Build history of the part. All positions in model axes, mm. Face numbers are marked on the shaded views. Give positions to 0.01 mm unless a question says otherwise; leave off trailing zeros. Write each loop counter-clockwise with the first axis right and the second up, starting at its lowest first coordinate (ties: lowest second). Pieces come first, ordered by that corner, then holes. Notation, with made-up numbers: (49, 58) -> (56, 58) arc R21 ccw to (56, 73) -> close; hole circle Ø10 at (70, -20). An arc over 180 degrees is marked (long way). Put each result on its own line as item: value.
from build123d import *

# Parameters (mm, degrees)
ESBO_O1_R                     = 2.25
RESSALTO_EXTRUS_O1_DEPTH      = 4
RESSALTO_EXTRUS_O2_DEPTH      = 10
RESSALTO_EXTRUS_O2_DEPTH_BACK = 4
ESBO_O2_W                     = 10
ESBO_O2_H                     = 20
ESBO_O2_R                     = 1.5
ESBO_O2_W_2                   = 3
FILETE1_R                     = 3
FILETE2_R                     = 3
FILETE3_R                     = 10
FILETE4_R                     = 10
FILETE6_R                     = 5
FILETE7_R                     = 5
FILETE8_R                     = 5


# Some blends are built 0.0001 mm under size
with BuildPart() as part:
    # Esboço1 → Ressalto-extrusão1 (new body)
    with BuildSketch(Plane.XY):
        with BuildLine():
            Line((30, 15.55), (30, 30.45))
            Line((30, 30.45), (30, 45.35))
            ThreePointArc((30, 45.35), (28.681980515, 48.531980515), (25.5, 49.85))
            Line((25.5, 49.85), (24.5, 49.85))
            Line((24.5, 49.85), (-26.5, 49.85))
            ThreePointArc((-26.5, 49.85), (-29.681980515, 48.531980515), (-31, 45.35))
            Line((-31, 45.35), (-31, 30.45))
            Line((-31, 30.45), (-31, 15.55))
            ThreePointArc((-31, 15.55), (-29.681980515, 12.368019485), (-26.5, 11.05))
            Line((-26.5, 11.05), (25.5, 11.05))
            ThreePointArc((25.5, 11.05), (28.681980515, 12.368019485), (30, 15.55))
        make_face()
        with Locations((-24.8, 25.45)):
            Circle(ESBO_O1_R, mode=Mode.SUBTRACT)
        with Locations((23.8, 25.45)):
            Circle(ESBO_O1_R, mode=Mode.SUBTRACT)
        with Locations((-24.8, 35.45)):
            Circle(ESBO_O1_R, mode=Mode.SUBTRACT)
        Polygon((27, 31.05), (27, 30.45), (27, 29.85), (20, 29.85), (20, 20.45), (-21, 20.45), (-21, 29.85), (-28, 29.85), (-28, 31.05), (-21, 31.05), (-21, 40.45), (20, 40.45), (20, 31.05), align=None, mode=Mode.SUBTRACT)
        with Locations((23.8, 35.45)):
            Circle(ESBO_O1_R, mode=Mode.SUBTRACT)
    extrude(amount=RESSALTO_EXTRUS_O1_DEPTH)

    # Esboço2 → Ressalto-extrusão2 (add, two sides: drawn at the far end of the back side and taken through both)
    # profile 1 of 5: a face of its own
    with BuildSketch(Plane.XY.offset(4).offset(-RESSALTO_EXTRUS_O2_DEPTH_BACK)):
        with Locations((-0.6, 59.85)):
            Rectangle(ESBO_O2_W, ESBO_O2_H)
        with Locations((-1.6, 54.35)):
            Circle(ESBO_O2_R, mode=Mode.SUBTRACT)
        with Locations((-1.6, 63.85)):
            Circle(ESBO_O2_R, mode=Mode.SUBTRACT)
    # profile 2 of 5: a face of its own
    with BuildSketch(Plane.XY.offset(4).offset(-RESSALTO_EXTRUS_O2_DEPTH_BACK)):
        with Locations((5.9, 59.85)):
            Rectangle(ESBO_O2_W_2, ESBO_O2_H)
    # profile 3 of 5: a face of its own
    with BuildSketch(Plane.XY.offset(4).offset(-RESSALTO_EXTRUS_O2_DEPTH_BACK)):
        Polygon((30, 32.45), (30, 30.45), (30, 28.45), (55, 28.45), (55, 32.45), align=None)
    # profile 4 of 5: a face of its own
    with BuildSketch(Plane.XY.offset(4).offset(-RESSALTO_EXTRUS_O2_DEPTH_BACK)):
        with Locations((-0.6, 1.05)):
            Rectangle(ESBO_O2_W, ESBO_O2_H)
        with Locations((-1.6, -2.95)):
            Circle(ESBO_O2_R, mode=Mode.SUBTRACT)
        with Locations((-1.6, 6.55)):
            Circle(ESBO_O2_R, mode=Mode.SUBTRACT)
    # profile 5 of 5: a face of its own
    with BuildSketch(Plane.XY.offset(4).offset(-RESSALTO_EXTRUS_O2_DEPTH_BACK)):
        with Locations((5.9, 1.05)):
            Rectangle(ESBO_O2_W_2, ESBO_O2_H)
    extrude(amount=RESSALTO_EXTRUS_O2_DEPTH + RESSALTO_EXTRUS_O2_DEPTH_BACK)

    # Filete1
    filete1_edges = [part.edges().sort_by_distance(p)[0] for p in [
        (30, 30.45, 4),
    ]]
    fillet(filete1_edges, radius=FILETE1_R - 0.0001)  # a hair under: the kernel refuses the full size

    # Filete2
    filete2_edges = [part.edges().sort_by_distance(p)[0] for p in [
        (30, 30.45, 14),
    ]]
    fillet(filete2_edges, radius=FILETE2_R)

    # Filete3
    # the kernel refuses this fillet: 10 mm, written as the material it adds along each edge
    with BuildSketch(Plane(origin=(-5.6, 11.05, 4), x_dir=(0, 1, 0), z_dir=(1, 0, 0))) as filete3_piece_1:
        with BuildLine():
            CenterArc((10, 9.981983771), FILETE3_R, 180, 86.560187232)
            Line((0, 9.981983771), (0, 0))
            Line((0, 0), (9.4, 0))
        make_face()
    extrude(amount=13)

    # Filete4
    # the kernel refuses this fillet: 10 mm, written as the material it adds along each edge
    with BuildSketch(Plane(origin=(-5.6, 49.85, 4), x_dir=(0, -1, 0), z_dir=(1, 0, 0))) as filete4_piece_1:
        with BuildLine():
            CenterArc((10, -9.981983771), FILETE4_R, 93.439812768, 86.560187232)
            Line((0, -9.981983771), (0, 0))
            Line((0, 0), (9.4, 0))
        make_face()
    extrude(amount=13)

    # Filete6
    # the kernel refuses this fillet: 5 mm, written as the material it takes off along each edge
    with BuildSketch(Plane(origin=(-18.1, 69.85, 0), x_dir=(0, -1, 0), z_dir=(1, 0, 0))) as filete6_piece_1:
        with BuildLine():
            CenterArc((FILETE6_R, -FILETE6_R), FILETE6_R, 90, 90)
            Line((0, -FILETE6_R), (0, 0))
            Line((0, 0), (FILETE6_R, 0))
        make_face()
    extrude(amount=38, mode=Mode.SUBTRACT)

    # Filete7
    # the kernel refuses this fillet: 5 mm, written as the material it takes off along each edge
    with BuildSketch(Plane(origin=(19.9, -8.95, 0), x_dir=(0, 1, 0), z_dir=(-1, 0, 0))) as filete7_piece_1:
        with BuildLine():
            CenterArc((FILETE7_R, -FILETE7_R), FILETE7_R, 90, 90)
            Line((0, -FILETE7_R), (0, 0))
            Line((0, 0), (FILETE7_R, 0))
        make_face()
    extrude(amount=38, mode=Mode.SUBTRACT)

    # Filete8
    filete8_edges = [part.edges().sort_by_distance(p)[0] for p in [
        (55, 30.45, 0),
    ]]
    fillet(filete8_edges, radius=FILETE8_R)


solid = part.part
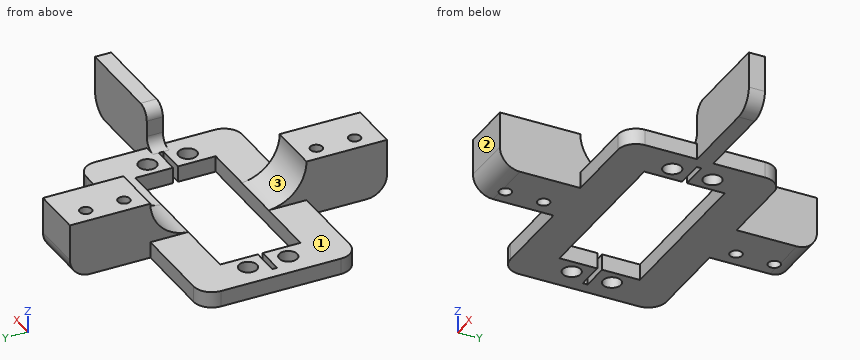
1) Slice it at A-A (x = -24.8). Write the cut outline in (y, z), plus the area to 3 significant figures.
Filled sheet:
outline: (11.05, 0) -> (23.2, 0) -> (23.2, 4) -> (11.05, 4) -> close; (27.7, 0) -> (29.85, 0) -> (29.85, 4) -> (27.7, 4) -> close; (31.05, 0) -> (33.2, 0) -> (33.2, 4) -> (31.05, 4) -> close; (37.7, 0) -> (49.85, 0) -> (49.85, 4) -> (37.7, 4) -> close
area: 114 mm2
2) Slice it at D-D (x = 11). Write the cut outline in (y, z), plus the area to 3 significant figures.
Filled sheet:
outline: (11.05, 0) -> (20.45, 0) -> (20.45, 4) -> (11.05, 4) -> close; (40.45, 0) -> (49.85, 0) -> (49.85, 4) -> (40.45, 4) -> close
area: 75.2 mm2
3) Pull direction Y, two halves, no side cores. Call the marked faces 1, 2 and 3: released by +Y, released by -Y, zero draft, split by the parting line, or undercut.
Filled sheet:
face 1: zero draft
face 2: released by -Y
face 3: undercut
4) Pin check, flat tips, straight feed: pin 1 (4 mm diameter, centred on x = 42.5, z = 8, fed in from +Y); pin 2 (1.2 mm diameter, centred on x = 9.5, z = 1, fed in from -Y); pin 3 (1.2 mm diameter, centred on x = -1, z = 2.5, fed in from +Y); pin 4 (3.5 mm diameter, centred on x = -24.8, y = 35.45, fed in from +Z). Stop position of each tip, or through.
Filled sheet:
pin 1: y = 32.45
pin 2: y = 11.05
pin 3: y = 69.47
pin 4: through
5) Wall check: L1, parallel to Y at x = -24.8, z = 2.25; L2, parallel to Y at x = -1.6, z = 6.5; L3, parallel to Y at x = -1.6, z = 9.5. Give the ranges that are in metal, low to high.
Filled sheet:
L1: 11.05 to 23.2, 27.7 to 29.85, 31.05 to 33.2, 37.7 to 49.85
L2: -8.95 to -4.45, -1.45 to 5.05, 8.05 to 14.42, 46.48 to 52.85, 55.85 to 62.35, 65.35 to 69.85
L3: -8.95 to -4.45, -1.45 to 5.05, 8.05 to 12.11, 48.79 to 52.85, 55.85 to 62.35, 65.35 to 69.85
6) Slice it at C-C (y = 63.85). Write the cut outline in (x, z), plus the area to 3 significant figures.
Filled sheet:
outline: (-5.6, 0) -> (-3.1, 0) -> (-3.1, 14) -> (-5.6, 14) -> close; (-0.1, 0) -> (7.4, 0) -> (7.4, 14) -> (-0.1, 14) -> close
area: 140 mm2
7) Slice it at B-B (z = 9.5). Write the cut outline in (x, y), plus the area to 3 significant figures.
Filled sheet:
outline: (-5.6, -8.95) -> (7.4, -8.95) -> (7.4, 12.11) -> (-5.6, 12.11) -> close; (-5.6, 48.79) -> (7.4, 48.79) -> (7.4, 69.85) -> (-5.6, 69.85) -> close; (30, 28.45) -> (55, 28.45) -> (55, 32.45) -> (30, 32.45) -> close; hole circle Ø3 at (-1.6, -2.95); hole circle Ø3 at (-1.6, 6.55); hole circle Ø3 at (-1.6, 54.35); hole circle Ø3 at (-1.6, 63.85)
area: 619 mm2
